Source: CAD feature listing. Evaluate the final solid. Frame: model axes, mm. Give positions to 0.01 mm unless a question says otherwise; leave off trailing zeros. Write each loop counter-clockwise with the first axis right and the second up, starting at its lowest first coordinate (ties: lowest second). Pieces come first, ordered by that corner, then holes. Notation, with made-up numbers: (40.25, 46) -> (73.25, 46) arc R28 cw to (73.25, 70) -> close; hole circle Ø8 at (38, -25). An arc over 180 degrees is marked (long way). Write item = value, one per line.
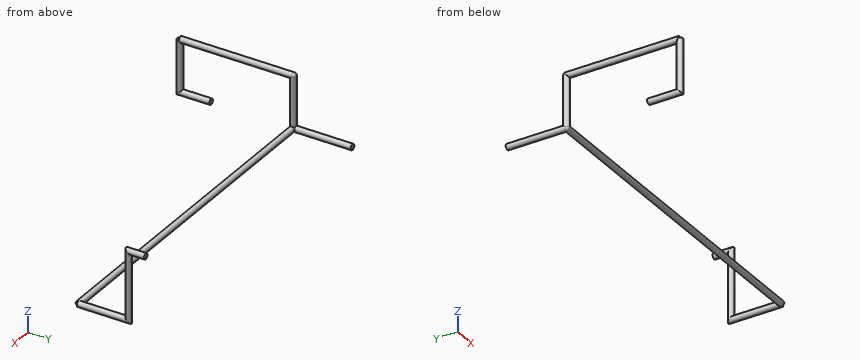
from build123d import *

# Parameters (mm, degrees)
F0_R  = 7.5
F5_R  = 7.5
F7_R  = 7.5
F10_R = 7.5
F15_R = 7.5
F19_R = 7.5


with BuildPart() as f2:
    # F2: sweep along a path in F1
    with BuildLine(Plane.YZ) as f2_path:
        Line((0, 0), (-80.781, 0))
        Line((-80.781, 0), (-80.781, 134.381))
    # F0 (on Front) → F2 (sweep)
    with BuildSketch(Plane.XZ):
        Circle(F0_R)
    sweep(path=f2_path.line, transition=Transition.RIGHT)



with BuildPart() as f6:
    # F6: sweep along a path in F3
    with BuildLine(Plane.XY) as f6_path:
        Line((0, 276.3272254467), (0, 123.3272254467))
    # F5 (on offset) → F6 (sweep)
    with BuildSketch(Plane.XZ.offset(-366)):
        Circle(F5_R)
    sweep(path=f6_path.line)

    # F8: sweep along a path in F1
    with BuildLine(Plane.YZ) as f8_path:
        Line((-80.781, 0), (-80.781, 134.381))
    # F7 (on Top) → F8 (sweep)
    with BuildSketch(Plane.XY):
        with Locations((0, 213)):
            Circle(F7_R)
    sweep(path=f8_path.line)


with BuildPart() as f2_1:
    add(f2.part)

    add(f6.part)  # F12 merges F6
    # F12: sweep along a path in F11
    with BuildLine(Plane.YZ) as f12_path:
        Line((211.219, 134.381), (-80.781, 134.381))
    # F10 (on offset) → F12 (sweep)
    with BuildSketch(Plane.XZ.offset(-213)):
        with Locations((0, 134.381)):
            Circle(F10_R)
    sweep(path=f12_path.line)

    # F8_face (on face) → F13 (revolve)
    with BuildSketch(Plane(origin=(0, 216.1830988618, 134.381), x_dir=(1, 0, 0), z_dir=(0, 0, 1))):
        with BuildLine():
            Line((-7.5, -3.1830988618), (7.5, -3.1830988618))
            ThreePointArc((7.5, -3.1830988618), (0, 4.3169011382), (-7.5, -3.1830988618))
        make_face()
    revolve(axis=Axis((0, 213, 134.381), (-1, 0, 0)))

    # F8_face1 (on face) → F14 (revolve)
    with BuildSketch(Plane(origin=(0, 209.8169011382, 0), x_dir=(1, 0, 0), z_dir=(0, 0, -1))):
        with BuildLine():
            ThreePointArc((7.5, -3.1830988618), (0, 4.3169011382), (-7.5, -3.1830988618))
            Line((-7.5, -3.1830988618), (7.5, -3.1830988618))
        make_face()
    revolve(axis=Axis((0, 213, 0), (1, 0, 0)))

    # F17: sweep along a path in F16
    with BuildLine(Plane.XZ.offset(-213)) as f17_path:
        Line((0, 0), (887.5, 0))
    # F15 (on Right) → F17 (sweep)
    with BuildSketch(Plane.YZ):
        with Locations((213, 0)):
            Circle(F15_R)
    sweep(path=f17_path.line)

    # F20: sweep along a path in F18
    with BuildLine(Plane.YZ) as f20_path:
        Line((213, 0), (343, 0))
        Line((343, 0), (343, 176))
        Line((343, 176), (386.726, 176))
    # F19 (on offset) → F20 (sweep)
    with BuildSketch(Plane.XZ.offset(-213)):
        with Locations((887.5, 0)):
            Circle(F19_R)
    sweep(path=f20_path.line, transition=Transition.RIGHT)


solid = f2_1.part
1) Cut plane C-C (x = 172). Return the cut outline in (y, z).
Computed:
outline = circle Ø15 at (213, 0)
2) Cut plane A-A (y = -44). Return the cut outline in (x, z), then the cut area to 3 significant figures.
Computed:
outline = circle Ø15 at (0, 0); circle Ø15 at (0, 134.38)
area = 353 mm²
3) Cut plane B-B (z = 103.5). Return the cut outline in (x, y).
Computed:
outline = circle Ø15 at (0, -80.78); circle Ø15 at (0, 213); circle Ø15 at (887.5, 343)
4) Contact query for flat-ended pins moving along their axis: pin 1 (7.5 mm diameter, centred on x = -3.5, z = -1.5, fed in from +Y); pin 2 (4.5 mm diameter, centred on x = -1.5, z = 138, fed in from -Y); pin 3 (7.5 mm diameter, centred on x = -2, y = -83.5, fed in from +Z). Output: stop coordinate, or through.
Computed:
pin_1 = 366
pin_2 = -79
pin_3 = 134.38
5) Material intervals for L1, parallel to Y at x = 704.5, z = 2, sorted ascending.
Computed:
L1 = 205.77 to 220.23
6) Cut plane D-D (y = 76). Return the cut outline in (x, z).
Computed:
outline = circle Ø15 at (0, 134.38)
